```python
from build123d import *

# Parameters (mm, degrees)
SKETCH_1_R          = 35
SKETCH_1_R_2        = 20
EXTRUDE_1_DEPTH     = 6
SKETCH_2_R          = 2.15
CUT_EXTRUDE_1_DEPTH = 70
FILLET_2_R          = 2
SKETCH_3_R          = 23.4
SKETCH_3_R_2        = 20
EXTRUDE_2_DEPTH     = 2


with BuildPart() as part:
    # 草图1 → 凸台-拉伸1 (new body)
    with BuildSketch(Plane(origin=(0, 0, 0), x_dir=(1, 0, 0), z_dir=(0, 1, 0))):
        with Locations(Location((0, 0, 0), (0, 0, 270))):
            Circle(SKETCH_1_R)
        with Locations(Location((0, 0, 0), (0, 0, 270))):
            Circle(SKETCH_1_R_2, mode=Mode.SUBTRACT)
    extrude(amount=EXTRUDE_1_DEPTH)

    # 草图2 → 切除-拉伸1 (cut)
    with BuildSketch(Plane(origin=(0, 6, 0), x_dir=(1, 0, 0), z_dir=(0, 1, 0))):
        with Locations(Location((29, 0, 0), (0, 0, 270))):
            Circle(SKETCH_2_R)
        with Locations(Location((-14.5, -25.11473671, 0), (0, 0, 270))):
            Circle(SKETCH_2_R)
        with Locations(Location((-14.5, 25.11473671, 0), (0, 0, 270))):
            Circle(SKETCH_2_R)
    extrude(amount=-CUT_EXTRUDE_1_DEPTH, mode=Mode.SUBTRACT)

    # 圆角2
    fillet_2_edges = [part.edges().sort_by_distance(p)[0] for p in [
        (29, 0, -2.15),
        (-14.5, 0, 22.96473671),
        (-14.5, 0, -27.26473671),
    ]]
    fillet(fillet_2_edges, radius=FILLET_2_R)

    # 草图3 → 凸台-拉伸2 (add)
    with BuildSketch(Plane(origin=(0, 6, 0), x_dir=(1, 0, 0), z_dir=(0, 1, 0))):
        with Locations(Location((0, 0, 0), (0, 0, 270))):
            Circle(SKETCH_3_R)
        with Locations(Location((0, 0, 0), (0, 0, 270))):
            Circle(SKETCH_3_R_2, mode=Mode.SUBTRACT)
    extrude(amount=EXTRUDE_2_DEPTH)


solid = part.part
```
Here's how the part is built. I have some questions about the finished solid (model axes, mm). A direction names the side the tool comes from. Give positions to 0.01 mm unless a question says otherwise; leave off trailing zeros. Write each loop counter-clockwise with the first axis right and the second up, starting at its lowest first coordinate (ties: lowest second). Pieces come first, ordered by that corner, then holes. Notation, with made-up numbers: (50, 43) -> (104, 43) arc R20 cw to (104, 47) -> close; hole circle Ø9 at (73.25, 22). An arc over 180 degrees is marked (long way). Use one line per item in the form item = value.
1) If I drill on L1, parallel to X at y = 4.75, z = 0; L2, parallel to Y at x = 30, z = 15.5; L3, parallel to X at y = 7, z = -3, over which ranges is the centre line in solid material (lowest first)? Write a range as [from, to].
Verdict:
L1 = [-35, -20], [20, 26.85], [31.15, 35]
L2 = [0, 6]
L3 = [-23.21, -19.77], [19.77, 23.21]
2) Suppose I cut it at A-A (x = 0). Please give me the cut outline in (y, z), and give its area (3 significant figures).
Verdict:
outline = (0, -35) -> (6, -35) -> (6, -23.4) -> (8, -23.4) -> (8, -20) -> (0, -20) -> close; (0, 20) -> (8, 20) -> (8, 23.4) -> (6, 23.4) -> (6, 35) -> (0, 35) -> close
area = 194 mm2
3) Suppose I cut it at B-B (z = 0). Please give me the cut outline in (x, y).
Verdict:
outline = (-35, 0) -> (-20, 0) -> (-20, 8) -> (-23.4, 8) -> (-23.4, 6) -> (-35, 6) -> close; (20, 0) -> (24.85, 0) arc R2 ccw to (26.85, 2) -> (26.85, 6) -> (23.4, 6) -> (23.4, 8) -> (20, 8) -> close; (31.15, 2) arc R2 ccw to (33.15, 0) -> (35, 0) -> (35, 6) -> (31.15, 6) -> close
4) I'm going to push flat-ended pins straight in: pin 1 (1 mm diameter, centred on y = 3, z = -26, fed in from -X); pin 2 (5.5 mm diameter, centred on x = 29, z = 0, fed in from +Y); pin 3 (1.5 mm diameter, centred on x = -4.5, y = 3.5, fed in from -Z). Where does each tip first touch, or does it pass through?
Verdict:
pin_1 = -23.97
pin_2 = 6
pin_3 = -34.8
5) We'd pull the mould along Z, two halves only. Please class faces 3 (the face through (11, 8, 17)), 4 (the face through (-21, 3, -28)), 5 (the face through (-19.524, 3.944, -4.336)): +Z half, -Z half, draft (parallel to the pull), parting line (faces both ways), or undercut.
Verdict:
face_3 = draft
face_4 = parting line
face_5 = undercut
6) Suppose I cut it at C-C (y = 3.25). Please give me the cut outline in (x, z).
Verdict:
outline = circle Ø70 at (0, 0); hole circle Ø40 at (0, 0); hole circle Ø4.3 at (-14.5, -25.11); hole circle Ø4.3 at (-14.5, 25.11); hole circle Ø4.3 at (29, 0)
7) On a 3-axis mill with a long thin cutter (end or side, diameter ignored), from which of +Z, -Z, +X, -X, +Y, -Y can I reach the whole of each face in a straight line? I mean faces 1 (the face through (-15, 0, 15)), 2 (the face through (-7, 6, 23)). Say none if no direction works.
Verdict:
face_1 = +Z, -Z, +X, -X, -Y
face_2 = +Y
8) Suppose I cut it at D-D (x = -14.5). Please give me the cut outline in (y, z), and give its area (3 significant figures).
Verdict:
outline = (0, -31.86) -> (6, -31.86) -> (6, -27.26) -> (2, -27.26) arc R2 ccw to (0, -29.26) -> close; (0, -20.96) arc R2 ccw to (2, -22.96) -> (6, -22.96) -> (6, -18.37) -> (8, -18.37) -> (8, -13.77) -> (0, -13.77) -> close; (0, 13.77) -> (8, 13.77) -> (8, 18.37) -> (6, 18.37) -> (6, 22.96) -> (2, 22.96) arc R2 ccw to (0, 20.96) -> close; (0, 29.26) arc R2 ccw to (2, 27.26) -> (6, 27.26) -> (6, 31.86) -> (0, 31.86) -> close
area = 180 mm2
